For this review, take the finished solid that the model builds, in its own axes (mm). Face numbers are marked on the shaded views. Coordinates: 2 decimals unless noted, no trailing zeros. Order: outer loops, then holes, each group sorted by start corner. A loop starts at its lowest first (then second) coordinate and runs counter-clockwise, first axis right, second up. Notation, with made-up numbers: (44.5, 84) -> (70.5, 84) arc R33 ccw to (70.5, 112) -> close; hole circle Ø8 at (41.5, -31). An arc over 180 degrees is marked (long way). Write item = value, one per line. Start each with the question number.
1) Consider section A-A on z = 37.5. Give the boundary of the cut face in (x, y) (3 decimals).
2) Consider section C-C on y = -2.25. Give the boundary of the cut face in (x, z).
3) Consider section B-B on x = 0. Give the boundary of the cut face in (y, z) (3 decimals), and give its area (3 significant figures).
4) Draft analysis for pull direction Y (two halves, no side actions). For the marked faces 1, 2 and 3, state which applies: +Y half, -Y half, draft (parallel to the pull), parting line (faces both ways), or undercut.
5) Wall thickness on probe 1 along Y at (x, z) = (0, 3.65); probe 2 along Y at (x, z) = (0, 38.5) (3 decimals); probe 3 along X at (y, z) = (-0.25, 40.5): over which ranges is each line inside the solid? List them lowest first. Write a range as [from, to].
6) Insertion check: pin 1 Ø7 at (x, y) = (0, 0) entering from +Z; pin 2 Ø3 at (x, y) = (-2.5, 0.5) entering from +Z; pin 3 Ø8 at (x, y) = (2.5, 2) entering from -Z. Each pin has a flat end and moves straight along its axis. Give the tip position at first contact, or say it passes through.
Autodesk Inventor part; units mm, degrees
ref_plane "YZ Plane" through (0, 0, 0) normal (1, 0, 0) x (0, 1, 0)
ref_plane "XZ Plane" through (0, 0, 0) normal (0, 1, 0) x (-1, 0, 0)
ref_plane "XY Plane" through (0, 0, 0) normal (0, 0, 1) x (1, 0, 0)
sketch "Sketch1" plane through (0, 0, 0) normal (0, 0, 1) x (1, 0, 0)
  line L0 (-8, 8) -> (8, 8)
  line L1 (8, 8) -> (8, -8)
  line L2 (8, -8) -> (-8, -8)
  line L3 (-8, -8) -> (-8, 8)
  line L4 (-8, 8) -> (8, -8) construction
  line L5 (8, 8) -> (-8, -8) construction
  point P0 (0, 0)
  dimension "d0" = 16
  dimension "d1" = 16
extrude "Extrusion1" add sketch "Sketch1" along normal blind 63.5
sketch "Sketch2" plane through (0, 0, 63.5) normal (0, 0, 1) x (1, 0, 0)
  circle A0 centre (0, 0) radius 5.075
  dimension "d4" = 10.15
extrude "Extrusion2" cut sketch "Sketch2" against normal blind 58.5
sketch "Sketch3" plane through (0, 0, 5) normal (0, 0, 1) x (1, 0, 0)
  circle A0 centre (0, 0) radius 4
  dimension "d7" = 8
extrude "Extrusion3" cut sketch "Sketch3" against normal up to surface (5 mm away)
properties part number "holder"
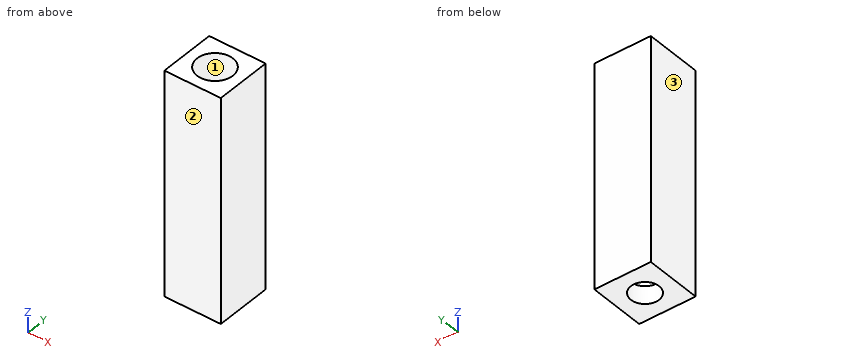
Answer sheet:
q1.outline = (-8, -8) -> (8, -8) -> (8, 8) -> (-8, 8) -> close; hole circle Ø10.15 at (0, 0)
q2.outline = (-8, 0) -> (-3.31, 0) -> (-3.31, 5) -> (-4.55, 5) -> (-4.55, 63.5) -> (-8, 63.5) -> close; (3.31, 0) -> (8, 0) -> (8, 63.5) -> (4.55, 63.5) -> (4.55, 5) -> (3.31, 5) -> close
q3.outline = (-8, 0) -> (-4, 0) -> (-4, 5) -> (-5.075, 5) -> (-5.075, 63.5) -> (-8, 63.5) -> close; (4, 0) -> (8, 0) -> (8, 63.5) -> (5.075, 63.5) -> (5.075, 5) -> (4, 5) -> close
q3.area = 382 mm2
q4.face_1 = undercut
q4.face_2 = -Y half
q4.face_3 = draft
q5.probe_1 = [-8, -4], [4, 8]
q5.probe_2 = [-8, -5.075], [5.075, 8]
q5.probe_3 = [-8, -5.07], [5.07, 8]
q6.pin_1 = through
q6.pin_2 = 5
q6.pin_3 = 0
